Can you work these out from the model? Positions are in its coordinate system, mm. Round coordinates to 2 decimals unless told otherwise and drop trailing zeros. Write each loop counter-clockwise with the first axis right and the second up, starting at its lowest first coordinate (ties: lowest second). Pieces come first, ordered by that corner, then holes. Notation, with made-up numbers: M 34.5,-21 L 66.5,-21 A26 ccw 66.5,5 Z; hole C -38.75,71 d1. An arc over 180 degrees is marked long. Answer in a Markdown table with one row per item. Add a question column.
(1) Suppose I cut it at C-C, the plane z = -65.5. Write out the boundary of the cut face in (x, y).
(2) I'm going to push flat-ended pins straight in: pin 1 (1 mm diameter, centred on x = 219.5, y = -39, fed in from -Z); pin 2 (10 mm diameter, centred on x = 18.5, z = -59.5, fed in from +Y); pin 3 (10 mm diameter, centred on x = -1, z = -61, fed in from +Y). Where does each tip first touch, or does it pass through?
(3) Suppose I cut it at A-A, the plane x = -201.5. Write out the boundary of the cut face in (y, z).
(4) If I drill on probe 1 along Y at (x, z) = (-162.5, -68.5); probe 2 along Y at (x, z) = (-43, -57); probe 3 along Z at (x, y) = (180.5, 53.5), over which ranges is the centre line in solid material (lowest first)?
(5) Suppose I cut it at B-B, the plane y = 55. Write out the boundary of the cut face in (x, z), then the cut area to 3 significant figures.
from build123d import *

# Parameters (mm, degrees)
BOSS_EXTRUDE1_DEPTH = 304.8


with BuildPart() as part:
    # Sketch1 → Boss-Extrude1 (new, symmetric)
    with BuildSketch(Plane(origin=(0, 0, 0), x_dir=(0, 0, -1), z_dir=(1, 0, 0))):
        with BuildLine():
            Line((49.373646209, 66.02166065), (-1.426353791, 66.02166065))
            Line((-1.426353791, 66.02166065), (-1.426353791, -60.97833935))
            Line((-1.426353791, -60.97833935), (49.373646209, -60.97833935))
            ThreePointArc((49.373646209, -60.97833935), (71.824286512, -51.678979653), (81.123646209, -29.22833935))
            Line((81.123646209, -29.22833935), (81.123646209, 34.27166065))
            ThreePointArc((81.123646209, 34.27166065), (71.824286512, 56.722300952), (49.373646209, 66.02166065))
        make_face()
    extrude(amount=BOSS_EXTRUDE1_DEPTH, both=True)


solid = part.part
Calculated:
| question | item | result |
|---|---|---|
| 1 | outline | M -304.8,-56.58 L 304.8,-56.58 L 304.8,61.62 L -304.8,61.62 Z |
| 2 | pin 1 | z = -79.74 |
| 2 | pin 2 | y = 65.61 |
| 2 | pin 3 | y = 65.32 |
| 3 | outline | M -60.98,-49.37 A31.75 ccw -29.23,-81.12 L 34.27,-81.12 A31.75 ccw 66.02,-49.37 L 66.02,1.43 L -60.98,1.43 Z |
| 4 | probe 1 | -54.57 to 59.61 |
| 4 | probe 2 | -60.05 to 65.09 |
| 4 | probe 3 | -74.64 to 1.43 |
| 5 | outline | M -304.8,-73.42 L 304.8,-73.42 L 304.8,1.43 L -304.8,1.43 Z |
| 5 | area | 45,600 mm² |
